from build123d import *

# Parameters (mm, degrees)
SKETCH1_R          = 5
BASE_EXTRUDE_DEPTH = 10


with BuildPart() as part:
    # Sketch1 → Base-Extrude (new body)
    with BuildSketch(Plane.XY):
        Polygon((0, 0), (25, 0), (175, 75), (175, 100), (0, 100), align=None)
        with Locations((12.5, 12.5)):
            Circle(SKETCH1_R, mode=Mode.SUBTRACT)
        with Locations((12.5, 87.5)):
            Circle(SKETCH1_R, mode=Mode.SUBTRACT)
        with BuildLine():
            Line((50, 50.159053651), (50, 69))
            ThreePointArc((50, 69), (51.757359313, 73.242640687), (56, 75))
            Line((56, 75), (93.681892698, 75))
            ThreePointArc((93.681892698, 75), (99.521386634, 70.378517523), (96.365174271, 63.633436854))
            Line((96.365174271, 63.633436854), (58.683281573, 44.792490505))
            ThreePointArc((58.683281573, 44.792490505), (52.845613327, 45.055148801), (50, 50.159053651))
        make_face(mode=Mode.SUBTRACT)
    extrude(amount=BASE_EXTRUDE_DEPTH)


solid = part.part
Geometry check sheet. Reference: the model listing, model coordinates, mm. A direction names the side the tool comes from. Round coordinates to 2 decimals unless told otherwise and drop trailing zeros. Write each loop counter-clockwise with the first axis right and the second up, starting at its lowest first coordinate (ties: lowest second). Pieces come first, ordered by that corner, then holes. Notation, with made-up numbers: (-12.5, 24.5) - (29.5, 24.5) arc R24 ccw to (29.5, 51.5) - close; hole circle Ø10 at (69.5, 29). An arc over 180 degrees is marked (long way). One line per item, written item: value.
1. Cross-section at B-B on x = 12.5. Record the boundary of the cut face in (y, z).
The answers:
outline: (0, 0) - (7.5, 0) - (7.5, 10) - (0, 10) - close; (17.5, 0) - (82.5, 0) - (82.5, 10) - (17.5, 10) - close; (92.5, 0) - (100, 0) - (100, 10) - (92.5, 10) - close
2. Cross-section at A-A on y = 87.5. Record the boundary of the cut face in (x, z), and give its area (3 significant figures).
The answers:
outline: (0, 0) - (7.5, 0) - (7.5, 10) - (0, 10) - close; (17.5, 0) - (175, 0) - (175, 10) - (17.5, 10) - close
area: 1,650 mm^2
3. Depth check by flat-ended pin: pin 1 Ø6 at (x, z) = (55, 6) entering from -Y; pin 2 Ø1.5 at (y, z) = (69.5, 4) entering from +X. Enter the tip coordinate at first touch or a pass-through.
The answers:
pin 1: stops at y = 13.5
pin 2: stops at x = 165.5
4. Set-up check for faces 5 (the face through (175, 87, 5)), 6 (the face through (51.711, 73.196, 4.93)): record each of +Z, -Z, +X, -X, +Y, -Y from which the full face is reachable in a straight line by a thin tool's end or side.
The answers:
face 5: +Z, -Z, +X, +Y, -Y
face 6: +Z, -Z
5. Cross-section at C-C on z = 5.75. Record the boundary of the cut face in (x, y).
The answers:
outline: (0, 0) - (25, 0) - (175, 75) - (175, 100) - (0, 100) - close; hole circle Ø10 at (12.5, 12.5); hole circle Ø10 at (12.5, 87.5); hole (50, 50.16) arc R6 ccw to (58.68, 44.79) - (96.37, 63.63) arc R6 ccw to (93.68, 75) - (56, 75) arc R6 ccw to (50, 69) - close
6. Mould release check, pull along X, two halves, no side actions. Record for faces 1 (the face through (99, 37, 5)), 2 (the face through (0, 51, 5)), 3 (the face through (89, 100, 5)), 4 (the face through (99.495, 70.488, 4.93)): released by +X, released by -X, zero draft, split by the parting line, or undercut.
The answers:
face 1: released by +X
face 2: released by -X
face 3: zero draft
face 4: undercut
7. Cross-section at D-D on x = 71. Record the boundary of the cut face in (y, z).
The answers:
outline: (23, 0) - (50.95, 0) - (50.95, 10) - (23, 10) - close; (75, 0) - (100, 0) - (100, 10) - (75, 10) - close
8. Scan lines: L1, parallel to Y at x = 12.5, z = 4; L2, parallel to X at y = 15.5, z = 6; L3, parallel to X at y = 22, z = 8. Record each from-to range of solid material in increasing order.
The answers:
L1: y = 0 to 7.5, 17.5 to 82.5, 92.5 to 100
L2: x = 0 to 8.5, 16.5 to 56
L3: x = 0 to 69
